Source: CAD feature listing. Evaluate the final solid. Frame: model axes, mm. A direction names the side the tool comes from. Give positions to 0.01 mm unless a question says otherwise; leave off trailing zeros. Write each loop counter-clockwise with the first axis right and the second up, starting at its lowest first coordinate (ties: lowest second). Pieces come first, ordered by that corner, then holes. Notation, with made-up numbers: (29, 23) -> (51, 23) arc R28 cw to (51, 46) -> close; hole circle Ø1 at (0, 64.5). An arc over 180 degrees is marked (long way). Write item = value, one per line.
from build123d import *

# Parameters (mm, degrees)
BOSS_EXTRUDE1_DEPTH         = 30
BOSS_EXTRUDE3_DEPTH         = 60
SKETCH8_R                   = 15.75
CUT_EXTRUDE3_DEPTH          = 30
CUT_EXTRUDE3_DRAFT          = -10
CIRPATTERN4_COPY_1_SKETCH_R = 15.75
CIRPATTERN4_COPY_1_DEPTH    = 30
CIRPATTERN4_COPY_1_DRAFT    = -10
CIRPATTERN4_COPY_2_SKETCH_R = 15.75
CIRPATTERN4_COPY_2_DEPTH    = 30
CIRPATTERN4_COPY_2_DRAFT    = -10
CIRPATTERN4_COPY_3_SKETCH_R = 15.75
CIRPATTERN4_COPY_3_DEPTH    = 30
CIRPATTERN4_COPY_3_DRAFT    = -10
CIRPATTERN4_COPY_4_SKETCH_R = 15.75
CIRPATTERN4_COPY_4_DEPTH    = 30
CIRPATTERN4_COPY_4_DRAFT    = -10
CIRPATTERN4_COPY_5_SKETCH_R = 15.75
CIRPATTERN4_COPY_5_DEPTH    = 30
CIRPATTERN4_COPY_5_DRAFT    = -10
CUT_EXTRUDE4_DEPTH          = 44
CIRPATTERN6_COUNT           = 6


with BuildPart() as part:
    # Sketch1 → Boss-Extrude1 (new body)
    with BuildSketch(Plane(origin=(0, 0, 0), x_dir=(1, 0, 0), z_dir=(0, 1, 0))):
        Polygon((40, -69.282032303), (80, 0), (40, 69.282032303), (-40, 69.282032303), (-80, 0), (-40, -69.282032303), align=None)
    extrude(amount=BOSS_EXTRUDE1_DEPTH)

    # Sketch2 → Boss-Extrude3 (add)
    with BuildSketch(Plane(origin=(0, 30, 0), x_dir=(1, 0, 0), z_dir=(0, 1, 0))):
        Polygon((20, -34.641016151), (40, 0), (20, 34.641016151), (-20, 34.641016151), (-40, 0), (-20, -34.641016151), align=None)
    extrude(amount=BOSS_EXTRUDE3_DEPTH)


with BuildPart() as cut_extrude3_tool:
    # Sketch8 → Cut-Extrude3 (with draft: the straight prism first)
    with BuildSketch(Plane(origin=(30, 0, 17.320508076), x_dir=(0.5000000000000001, 0, -0.8660254037844386), z_dir=(0.8660254037844386, 0, 0.5000000000000001))):
        with Locations((0, 60)):
            Circle(SKETCH8_R)
    extrude(amount=-CUT_EXTRUDE3_DEPTH)
    # Cut-Extrude3: the draft: its side faces are tilted about the plane it starts from
    cut_extrude3_sides = [cut_extrude3_tool.faces().sort_by_distance(p)[0] for p in [
        (9.134618943, 60, 23.460408185),
    ]]
    draft(cut_extrude3_sides, Plane(origin=(30, 0, 17.320508076), x_dir=(0.5000000000000001, 0, -0.8660254037844386), z_dir=(0.8660254037844386, 0, 0.5000000000000001)), CUT_EXTRUDE3_DRAFT)


with BuildPart() as part_1:
    add(part.part)

    # Cut-Extrude3: cut by cut_extrude3_tool
    add(cut_extrude3_tool.part, mode=Mode.SUBTRACT)


with BuildPart() as cirpattern4_copy_1_tool:
    # CirPattern4 copy 1 sketch → CirPattern4 copy 1 (with draft: the straight prism first)
    with BuildSketch(Plane(origin=(30, 0, -17.320508076), x_dir=(-0.4999999999999998, 0, -0.8660254037844388), z_dir=(0.8660254037844388, 0, -0.4999999999999998))):
        with Locations((0, 60)):
            Circle(CIRPATTERN4_COPY_1_SKETCH_R)
    extrude(amount=-CIRPATTERN4_COPY_1_DEPTH)
    # CirPattern4 copy 1: the draft: its side faces are tilted about the plane it starts from
    cirpattern4_copy_1_sides = [cirpattern4_copy_1_tool.faces().sort_by_distance(p)[0] for p in [
        (24.884618943, 60, 3.819392034),
    ]]
    draft(cirpattern4_copy_1_sides, Plane(origin=(30, 0, -17.320508076), x_dir=(-0.4999999999999998, 0, -0.8660254037844388), z_dir=(0.8660254037844388, 0, -0.4999999999999998)), CIRPATTERN4_COPY_1_DRAFT)


with BuildPart() as part_2:
    add(part_1.part)

    # CirPattern4 copy 1: cut by cirpattern4_copy_1_tool
    add(cirpattern4_copy_1_tool.part, mode=Mode.SUBTRACT)


with BuildPart() as cirpattern4_copy_2_tool:
    # CirPattern4 copy 2 sketch → CirPattern4 copy 2 (with draft: the straight prism first)
    with BuildSketch(Plane(origin=(0, 0, -34.641016151), x_dir=(-1, 0, 0), z_dir=(0, 0, -1))):
        with Locations((0, 60)):
            Circle(CIRPATTERN4_COPY_2_SKETCH_R)
    extrude(amount=-CIRPATTERN4_COPY_2_DEPTH)
    # CirPattern4 copy 2: the draft: its side faces are tilted about the plane it starts from
    cirpattern4_copy_2_sides = [cirpattern4_copy_2_tool.faces().sort_by_distance(p)[0] for p in [
        (15.75, 60, -19.641016151),
    ]]
    draft(cirpattern4_copy_2_sides, Plane(origin=(0, 0, -34.641016151), x_dir=(-1, 0, 0), z_dir=(0, 0, -1)), CIRPATTERN4_COPY_2_DRAFT)


with BuildPart() as part_3:
    add(part_2.part)

    # CirPattern4 copy 2: cut by cirpattern4_copy_2_tool
    add(cirpattern4_copy_2_tool.part, mode=Mode.SUBTRACT)


with BuildPart() as cirpattern4_copy_3_tool:
    # CirPattern4 copy 3 sketch → CirPattern4 copy 3 (with draft: the straight prism first)
    with BuildSketch(Plane(origin=(-30, 0, -17.320508076), x_dir=(-0.5000000000000002, 0, 0.8660254037844385), z_dir=(-0.8660254037844385, 0, -0.5000000000000002))):
        with Locations((0, 60)):
            Circle(CIRPATTERN4_COPY_3_SKETCH_R)
    extrude(amount=-CIRPATTERN4_COPY_3_DEPTH)
    # CirPattern4 copy 3: the draft: its side faces are tilted about the plane it starts from
    cirpattern4_copy_3_sides = [cirpattern4_copy_3_tool.faces().sort_by_distance(p)[0] for p in [
        (-9.134618943, 60, -23.460408185),
    ]]
    draft(cirpattern4_copy_3_sides, Plane(origin=(-30, 0, -17.320508076), x_dir=(-0.5000000000000002, 0, 0.8660254037844385), z_dir=(-0.8660254037844385, 0, -0.5000000000000002)), CIRPATTERN4_COPY_3_DRAFT)


with BuildPart() as part_4:
    add(part_3.part)

    # CirPattern4 copy 3: cut by cirpattern4_copy_3_tool
    add(cirpattern4_copy_3_tool.part, mode=Mode.SUBTRACT)


with BuildPart() as cirpattern4_copy_4_tool:
    # CirPattern4 copy 4 sketch → CirPattern4 copy 4 (with draft: the straight prism first)
    with BuildSketch(Plane(origin=(-30, 0, 17.320508076), x_dir=(0.4999999999999994, 0, 0.866025403784439), z_dir=(-0.866025403784439, 0, 0.4999999999999994))):
        with Locations((0, 60)):
            Circle(CIRPATTERN4_COPY_4_SKETCH_R)
    extrude(amount=-CIRPATTERN4_COPY_4_DEPTH)
    # CirPattern4 copy 4: the draft: its side faces are tilted about the plane it starts from
    cirpattern4_copy_4_sides = [cirpattern4_copy_4_tool.faces().sort_by_distance(p)[0] for p in [
        (-24.884618943, 60, -3.819392034),
    ]]
    draft(cirpattern4_copy_4_sides, Plane(origin=(-30, 0, 17.320508076), x_dir=(0.4999999999999994, 0, 0.866025403784439), z_dir=(-0.866025403784439, 0, 0.4999999999999994)), CIRPATTERN4_COPY_4_DRAFT)


with BuildPart() as part_5:
    add(part_4.part)

    # CirPattern4 copy 4: cut by cirpattern4_copy_4_tool
    add(cirpattern4_copy_4_tool.part, mode=Mode.SUBTRACT)


with BuildPart() as cirpattern4_copy_5_tool:
    # CirPattern4 copy 5 sketch → CirPattern4 copy 5 (with draft: the straight prism first)
    with BuildSketch(Plane.XY.offset(34.641016151)):
        with Locations((0, 60)):
            Circle(CIRPATTERN4_COPY_5_SKETCH_R)
    extrude(amount=-CIRPATTERN4_COPY_5_DEPTH)
    # CirPattern4 copy 5: the draft: its side faces are tilted about the plane it starts from
    cirpattern4_copy_5_sides = [cirpattern4_copy_5_tool.faces().sort_by_distance(p)[0] for p in [
        (-15.75, 60, 19.641016151),
    ]]
    draft(cirpattern4_copy_5_sides, Plane.XY.offset(34.641016151), CIRPATTERN4_COPY_5_DRAFT)


with BuildPart() as part_6:
    add(part_5.part)

    # CirPattern4 copy 5: cut by cirpattern4_copy_5_tool
    add(cirpattern4_copy_5_tool.part, mode=Mode.SUBTRACT)

    # Sketch3 → Cut-Extrude4 (cut)
    with BuildSketch(Plane(origin=(60, 0, 34.641016151), x_dir=(0.5000000000000001, 0, -0.8660254037844386), z_dir=(0.8660254037844386, 0, 0.5000000000000001))):
        with BuildLine():
            Line((-10, 25), (10, 25))
            ThreePointArc((10, 25), (20, 15), (10, 5))
            Line((10, 5), (-10, 5))
            ThreePointArc((-10, 5), (-20, 15), (-10, 25))
        make_face()
    cut_extrude4 = extrude(amount=-CUT_EXTRUDE4_DEPTH, mode=Mode.SUBTRACT)

    # CirPattern6: Cut-Extrude4 ×6 about axis
    cirpattern6_axis = Axis((0, 0, 0), (0, 1, 0))
    for i in range(1, CIRPATTERN6_COUNT):
        add(cut_extrude4.rotate(cirpattern6_axis, i * 360 / CIRPATTERN6_COUNT), mode=Mode.SUBTRACT)


solid = part_6.part
1) Contact query for flat-ended pins moving along their axis: pin 1 (1.6 mm diameter, centred on x = 0.5, y = 63, fed in from -Z); pin 2 (19.5 mm diameter, centred on x = -42, z = -30.5, fed in from +Y); pin 3 (3 mm diameter, centred on y = 12.5, z = 8, fed in from +X). Output: stop coordinate, or through.
Computed:
pin_1 = -4.64
pin_2 = 30
pin_3 = 76.25
2) Cut plane C-C (z = -54). Return the cut outline in (x, y), then the cut area to 3 significant figures.
Computed:
outline = (-48.82, 0) -> (48.82, 0) -> (48.82, 30) -> (-48.82, 30) -> close; hole (-10, 5) -> (10, 5) arc R10 ccw to (10, 25) -> (-10, 25) arc R10 ccw to start
area = 2,220 mm²
3) Access query for faces 5 (the cylindrical face through (20, 15, 48)), 6 (the flat face through (25.416, 46.247, 25.261)), 7 (the flat face through (-41, 5, 24)). Directions: +Z, -Z, +X, -X, +Y, -Y. A direction counts if a zero-diameter tool reaches every point of the face in a straight line with its end or side. Return the directions, or none.
Computed:
face_5 = +Z
face_6 = +Z, +X, +Y
face_7 = none
4) Draft query along Y for faces 1 (the flat face through (-41, 25, -24)), 2 (the conical face through (-20.224, 48.341, -4.674)), 3 (the flat face through (-9, 46, 34.641)), 4 (the flat face through (-1, 0, -1)). Return one class per face: pulls with the +Y half, pulls with the -Y half, needs draft (parallel to the pull), parting line crosses it, or undercut.
Computed:
face_1 = undercut
face_2 = undercut
face_3 = needs draft
face_4 = pulls with the -Y half
5) Cut plane D-D (y = 35.5). Return the cut outline in (x, z).
Computed:
outline = (-40, 0) -> (-20, -34.64) -> (20, -34.64) -> (40, 0) -> (20, 34.64) -> (-20, 34.64) -> close
6) Cut plane B-B (x = 0). Return the cut outline in (y, z).
Computed:
outline = (0, -69.28) -> (5, -69.28) -> (5, -25.28) -> (25, -25.28) -> (25, -69.28) -> (30, -69.28) -> (30, -34.64) -> (44.25, -34.64) -> (49.54, -4.64) -> (70.46, -4.64) -> (75.75, -34.64) -> (90, -34.64) -> (90, 34.64) -> (75.75, 34.64) -> (70.46, 4.64) -> (49.54, 4.64) -> (44.25, 34.64) -> (30, 34.64) -> (30, 69.28) -> (25, 69.28) -> (25, 25.28) -> (5, 25.28) -> (5, 69.28) -> (0, 69.28) -> close
7) Cut plane A-A (y = 60). State how many separate pieces and enclosed holes the cut face has, then the cut area to 3 significant figures.
Computed:
separate_pieces = 7
enclosed_holes = 0
area = 345 mm²
8) Material intervals for L1, parallel to Z at x = 50.5, y = 21; L2, parallel to Y at x = -29, z = 36.5; L3, parallel to Z at x = -12, y = 12, sorted ascending.
Computed:
L1 = -51.1 to -49.94, -8.37 to 8.37, 49.94 to 51.1
L2 = 0 to 7.97, 22.03 to 30
L3 = -25.28 to 25.28
